from build123d import *

# Parameters (mm, degrees)
BOSS_EXTRUDE1_DEPTH = 2
BOSS_EXTRUDE2_DEPTH = 4
CUT_EXTRUDE3_DEPTH  = 3.15
BOSS_EXTRUDE3_START = 0.5
BOSS_EXTRUDE3_DEPTH = 0.5
SKETCH8_R           = 2.1
CUT_EXTRUDE4_DEPTH  = 32.941352507


with BuildPart() as part:
    # Sketch1 → Boss-Extrude1 (new, symmetric)
    with BuildSketch(Plane.XY):
        with BuildLine():
            Line((16, 3), (-16, 3))
            ThreePointArc((-16, 3), (-25, 0), (-16, -3))
            Line((-16, -3), (16, -3))
            ThreePointArc((16, -3), (25, 0), (16, 3))
        make_face()
    extrude(amount=BOSS_EXTRUDE1_DEPTH, both=True)

    # Sketch3 → Boss-Extrude2 (add)
    with BuildSketch(Plane.XY.offset(2)):
        with BuildLine():
            ThreePointArc((-20.342845142, 6.991599045), (-27, 0), (-20.342845142, -6.991599045))
            Line((-20.342845142, -6.991599045), (15.124207365, -8.73078726))
            ThreePointArc((15.124207365, -8.73078726), (30, 0), (15.124207365, 8.73078726))
            Line((15.124207365, 8.73078726), (-20.342845142, 6.991599045))
        make_face()
        with BuildLine():
            ThreePointArc((-16, -3), (-25, 0), (-16, 3))
            Line((-16, 3), (16, 3))
            ThreePointArc((16, 3), (25, 0), (16, -3))
            Line((16, -3), (-16, -3))
        make_face(mode=Mode.SUBTRACT)
    extrude(amount=-BOSS_EXTRUDE2_DEPTH)

    # Sketch6 → Cut-Extrude3 (cut)
    with BuildSketch(Plane(origin=(0, 0, -2), x_dir=(-1, 0, 0), z_dir=(0, 0, -1))):
        with BuildLine():
            Line((-8, -3.5), (4, -3.5))
            ThreePointArc((4, -3.5), (7.5, 0), (4, 3.5))
            Line((4, 3.5), (-8, 3.5))
            ThreePointArc((-8, 3.5), (-12.021685318, 4.137122098), (-15.649519503, 5.986093838))
            ThreePointArc((-15.649519503, 5.986093838), (-27.4, 0), (-15.649519503, -5.986093838))
            ThreePointArc((-15.649519503, -5.986093838), (-12.021685318, -4.137122098), (-8, -3.5))
        make_face()
    extrude(amount=-CUT_EXTRUDE3_DEPTH, mode=Mode.SUBTRACT)

    # Sketch7 → Boss-Extrude3 (add)
    with BuildSketch(Plane.XY.offset(2).offset(BOSS_EXTRUDE3_START)):
        with BuildLine():
            ThreePointArc((-20.342845142, 6.991599045), (-27, 0), (-20.342845142, -6.991599045))
            ThreePointArc((-20.342845142, -6.991599045), (-15.172988295, -5.0695126), (-13, 0))
            ThreePointArc((-13, 0), (-15.172988295, 5.0695126), (-20.342845142, 6.991599045))
        make_face()
        with BuildLine():
            ThreePointArc((-13, 0), (-15.172988295, -5.0695126), (-20.342845142, -6.991599045))
            Line((-20.342845142, -6.991599045), (15.124207365, -8.73078726))
            ThreePointArc((15.124207365, -8.73078726), (10, 0), (15.124207365, 8.73078726))
            Line((15.124207365, 8.73078726), (-20.342845142, 6.991599045))
            ThreePointArc((-20.342845142, 6.991599045), (-15.172988295, 5.0695126), (-13, 0))
        make_face()
        with BuildLine():
            ThreePointArc((15.124207365, 8.73078726), (10, 0), (15.124207365, -8.73078726))
            ThreePointArc((15.124207365, -8.73078726), (25.061722713, -8.624323926), (30, 0))
            ThreePointArc((30, 0), (25.061722713, 8.624323926), (15.124207365, 8.73078726))
        make_face()
    extrude(amount=-BOSS_EXTRUDE3_DEPTH)

    # Sketch8 → Cut-Extrude4 (cut, through all)
    with BuildSketch(Plane(origin=(0, 0, -2), x_dir=(-1, 0, 0), z_dir=(0, 0, -1))):
        with Locations((20, 0)):
            Circle(SKETCH8_R)
    extrude(amount=-CUT_EXTRUDE4_DEPTH, mode=Mode.SUBTRACT)


solid = part.part
Work out the finished part from the listing and answer in its coordinate system (mm). A direction names the side the tool comes from. Round coordinates to 2 decimals unless told otherwise and drop trailing zeros. Write each loop counter-clockwise with the first axis right and the second up, starting at its lowest first coordinate (ties: lowest second). Pieces come first, ordered by that corner, then holes.
1) A cutting plane is placed at A-A (z = 0.4). Give the vertices of the cut face in (x, y).
2) A cutting plane is placed at D-D (y = 5). Give the vertices of the cut face in (x, z).
3) A tool of negligible diameter and unlimited length cuts with its end or side. For faces 1 (the cylindrical face through (-22.003, 0.631, 0.219)), 2 (the cylindrical face through (11.97, 4.12, -0.45)), from which of +Z, -Z, +X, -X, +Y, -Y can it reach the whole face along a straight path? Write none if from no direction.
4) The mould has two halves that part along Y. Classify faces 3 (the flat face through (2, 3.5, 0)), 4 (the flat face through (-2.361, 7.873, 0.281)), 5 (the cylindrical face through (-27, 0, 0)): pulls with the +Y half, pulls with the -Y half, needs draft (parallel to the pull), parting line crosses it, or undercut.
5) A cutting plane is placed at B-B (x = -19.5). Give the vertices of the cut face in (y, z).
6) Straight lines are drawn through the part: line 1 (Y direction, x = 20, z = 0.3); line 2 (X direction, y = -5, z = 0.1); line 3 (Y direction, x = 3.5, z = -1.6). For each, find the intervals that lie inside material, in ascending order.
7) A cutting plane is placed at C-C (x = 20). Give the vertices of the cut face in (y, z).
8) Given pin 1 Ø1 at (y, z) = (5.5, 1.5) entering from +X; pin 2 Ø1 at (x, z) = (13, -0.5) entering from -Y, each flat-ended and moving along its own axis, determine where each tip first touches the part or whether it passes through.
Completed:
1. outline: (-20.34, -6.99) - (15.12, -8.73) arc R10 ccw (long way) to (15.12, 8.73) - (-20.34, 6.99) arc R7 ccw to start; hole circle Ø4.2 at (-20, 0); hole (-4, -3.5) - (8, -3.5) arc R13.01 cw to (15.65, -5.99) arc R7.4 ccw (long way) to (15.65, 5.99) arc R13.01 cw to (8, 3.5) - (-4, 3.5) arc R3.5 ccw to start
2. outline: (-24.9, -2) - (14.07, -2) - (14.07, 1.15) - (25.46, 1.15) - (25.46, -2) - (28.66, -2) - (28.66, 2.5) - (-24.9, 2.5) - close
3. face 1: +Z, -Z
3. face 2: -Z
4. face 3: undercut
4. face 4: pulls with the +Y half
4. face 5: parting line crosses it
5. outline: (-7.03, -2) - (-2.04, -2) - (-2.04, 2.5) - (-7.03, 2.5) - close; (2.04, -2) - (7.03, -2) - (7.03, 2.5) - (2.04, 2.5) - close
6. line 1: y = -10 to -7.4, 7.4 to 10
6. line 2: x = -24.9 to 14.07, 25.46 to 28.66
6. line 3: y = -8.16 to -3.5, 3.5 to 8.16
7. outline: (-10, -2) - (-7.4, -2) - (-7.4, 1.15) - (7.4, 1.15) - (7.4, -2) - (10, -2) - (10, 2.5) - (-10, 2.5) - close
8. pin 1: stops at x = 28.66
8. pin 2: stops at y = -8.65
